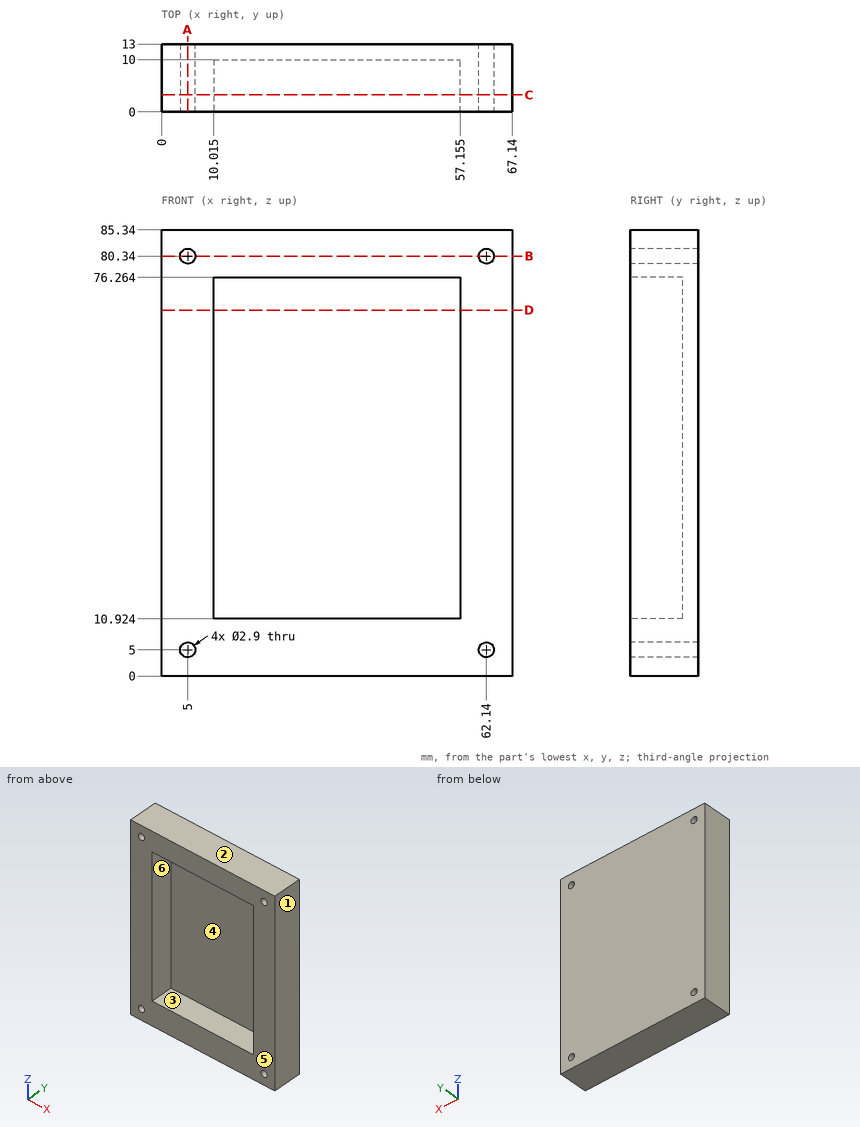
Geometry check sheet. Reference: drawing and pictorial views, mm from the part's lowest x, y, z. A direction names the side the tool comes from. Give positions to 0.01 mm unless a question says otherwise; leave off trailing zeros. Loops run counter-clockwise (first coordinate to the right, second up) from the corner with the lowest first, then second, coordinate; pieces in that order, holes last.
1. Thickness scan on line 1 (Z direction, x = 5, y = 8.75); line 2 (X direction, y = 9.5, z = 46) (1 decimal); line 3 (Z direction, x = 55.5, y = 8.25). Record the ranges inside material, lowest first.
2. Set-up check for the marked faces 5 and 6: record each of +Z, -Z, +X, -X, +Y, -Y from which the full face is reachable in a straight line by a thin tool's end or side.
3. Section check B-B, the plane z = 80.34. Enter the section's corners in (x, y).
4. Section check D-D, the plane z = 70. Enter the section's corners in (x, y) (1 decimal).
5. Mould release check, pull along X, two halves, no side actions. Record for the marked faces 1, 2, 3 and 4: released by +X, released by -X, zero draft, split by the parting line, or undercut.
6. Section check A-A, the plane x = 5. Enter the section's corners in (y, z), then the cut area to 3 significant figures.
7. Go/stop test with a flat-tipped pin: pin 1 Ø5 at (x, z) = (41, 31) entering from -Y. Record where the tip stops, or that it passes through.
8. Section check C-C, the plane y = 3.25. Count the separate pieces of the cut face and the enclosed holes in it, then the cut area to 3 significant figures.
Geometry says:
1. line 1: z = 0 to 3.55, 6.45 to 78.89, 81.79 to 85.34
1. line 2: x = 0 to 10, 57.2 to 67.1
1. line 3: z = 0 to 10.92, 76.26 to 85.34
2. face 5: +Z, -Z, +X, -X, -Y
2. face 6: -Y
3. outline: (0, 0) - (3.55, 0) - (3.55, 13) - (0, 13) - close; (6.45, 0) - (60.69, 0) - (60.69, 13) - (6.45, 13) - close; (63.59, 0) - (67.14, 0) - (67.14, 13) - (63.59, 13) - close
4. outline: (0, 0) - (10, 0) - (10, 10) - (57.2, 10) - (57.2, 0) - (67.1, 0) - (67.1, 13) - (0, 13) - close
5. face 1: released by +X
5. face 2: zero draft
5. face 3: undercut
5. face 4: undercut
6. outline: (0, 0) - (13, 0) - (13, 3.55) - (0, 3.55) - close; (0, 6.45) - (13, 6.45) - (13, 78.89) - (0, 78.89) - close; (0, 81.79) - (13, 81.79) - (13, 85.34) - (0, 85.34) - close
6. area: 1,030 mm2
7. pin 1: stops at y = 10
8. separate pieces: 1
8. enclosed holes: 5
8. area: 2,620 mm2
